Here's how the part is built. I have some questions about the finished solid (model axes, mm). A direction names the side the tool comes from. Coordinates: 2 decimals unless noted, no trailing zeros. Write each loop counter-clockwise with the first axis right and the second up, starting at its lowest first coordinate (ties: lowest second). Pieces come first, ordered by that corner, then holes. Notation, with made-up numbers: (-26, -29) -> (18, -29) arc R6 cw to (18, -21) -> close; hole circle Ø1 at (-23, 9). An arc over 180 degrees is marked (long way). Use a Markdown table: item, result. Add a question column.
Item 1: On a 3-axis mill with a long thin cutter (end or side, diameter ignored), from which of +Z, -Z, +X, -X, +Y, -Y can I reach the whole of each face in a straight line? I mean faces 1 (the cylindrical face through (3, 0, -1)), 2 (the cylindrical face through (-0.421, -0.434, 1.952)). Say none if no direction works.
Item 2: Will these pins go through, and if not, where does the flat tip stop? pin 1 Ø1.5 at (x, y) = (2, 0.5) entering from -Z; pin 2 Ø2 at (x, z) = (3, -0.5) entering from +Y; pin 3 Ø1.5 at (y, z) = (-1.5, 0) entering from +X.
Item 3: If we mould it in two halves opening along Y, with no side actions, what happens to faces 3 (the conical face through (0.558, -0.214, -0.964)), 4 (the flat face through (-0.83, 0, 0)), 5 (the flat face through (-1.6, 0.4, -0.7))? For each: pulls with the +Y half, pulls with the -Y half, needs draft (parallel to the pull), parting line crosses it, or undercut.
Item 4: If I drill on line 1 along Z through (x, y) = (4.75, 0); line 2 along Z through (x, y) = (4, 0.45), over which ranges is the centre line in solid material (lowest first)? Write a range as from..to.
Item 5: Imagine slicing it at A-A, the plane x = 0.25. Write out the boundary of the cut face in (y, z).
Autodesk Inventor part; units mm, degrees
ref_plane "YZ Plane" through (0, 0, 0) normal (1, 0, 0) x (0, 1, 0)
ref_plane "XZ Plane" through (0, 0, 0) normal (0, 1, 0) x (-1, 0, 0)
ref_plane "XY Plane" through (0, 0, 0) normal (0, 0, 1) x (1, 0, 0)
sketch "Sketch4" plane through (0, 0, 0) normal (0, 0, 1) x (1, 0, 0)
  line L0 (-1.6, 0) -> (6, 0)
  line L1 (0, 0) -> (-1.6, 0)
  line L2 (0, 2) -> (0, 1.38)
  line L3 (0.4, 0.98) -> (0.4, 0.98)
  line L4 (0.4, 0.98) -> (0.8, 1)
  arc A0 (0, 1.38) -> (0.4, 0.98) centre (0.4, 1.38) ccw
  line L5 (-1.6, 0) -> (-1.6, 1)
  line L6 (0, 2) -> (-0.83, 2)
  arc A1 (-0.83, 2) -> (-1.6, 1) centre (1.2707, -0.414) ccw
  line L7 (0.8, 1) -> (6, 1)
  line L8 (6, 1) -> (6, 0)
  point P0 (0, 0.98)
  dimension "d71" = 0.4
  dimension "d72" = 6
  dimension "d74" = 0.4
  dimension "d75" = 1.96
  dimension "d78" = 2
  dimension "d82" = 3.2
  dimension "d83" = 1.6
  dimension "d84" = 4
  dimension "d104" = 5.2
  dimension "d105" = 2
revolve "Revolution7" add sketch "Sketch4" angle 360 about axis through (-1.6, 0, 0) along (1, 0, 0)
sketch "Sketch5" plane through (-1.6, 0, 0) normal (-1, 0, 0) x (0, 0, 1)
  circle A0 centre (0, 0) radius 0.875 construction
  circle A1 centre (0, 0) radius 0.6125 construction
  line L0 (0, 0) -> (-0.5304, 0.3062)
  line L1 (0, 0) -> (-0.5304, -0.3063)
  line L2 (-1.8008, 0) -> (1.7887, 0)
  line L3 (-0.875, 0) -> (-0.5304, -0.3063)
  line L4 (-0.875, 0) -> (-0.5304, 0.3062)
  point P0 (0, 0)
  dimension "d88" = 1.75
  dimension "d89" = 1.225
  dimension "d90" = 30
  dimension "d91" = 30
extrude "Extrusion1" cut sketch "Sketch5" against normal blind 0.77
pattern_circular "Circular Pattern1" count 6 over 360 about axis through (-10, 0, 0) along (1, 0, 0) of "Extrusion1"
fillet "Fillet1" radius 0.175 12 edges at (-1.215, -0.7578, -0.4375) (-1.215, -0.3063, -0.5304) (-1.215, -0.6125, 0) (-1.215, -0.7578, 0.4375) (-1.215, -0.3062, 0.5304) (-1.215, 0, 0.875) (-1.215, 0.6125, 0) (-1.215, 0.7578, 0.4375) (-1.215, 0.3063, 0.5304) (-1.215, 0.3062, -0.5304) (-1.215, 0, -0.875) (-1.215, 0.7578, -0.4375)
thread "Thread7"
properties part number "Šroub s válcovou hlavou a šestiramennou drážkou ISO 14583 - M2 x 6 - 4.8" material "Steel"
Ans:
| question | item | result |
|---|---|---|
| 1 | face 1 | +X |
| 1 | face 2 | +X, -X |
| 2 | pin 1 | stops at z = -1 |
| 2 | pin 2 | stops at y = 1 |
| 2 | pin 3 | stops at x = 6 |
| 3 | face 3 | parting line crosses it |
| 3 | face 4 | undercut |
| 3 | face 5 | needs draft |
| 4 | line 1 | z = -1..1 |
| 4 | line 2 | z = -0.89..0.89 |
| 5 | outline | circle Ø2.02 at (0, 0) |
